Design review of the part built by this model. Coordinates are the model's own, in mm. Give positions to 0.01 mm unless a question says otherwise; leave off trailing zeros. Write each loop counter-clockwise with the first axis right and the second up, starting at its lowest first coordinate (ties: lowest second). Pieces come first, ordered by that corner, then holes. Notation, with made-up numbers: (2.25, 6.25) -> (29.25, 6.25) arc R12 ccw to (29.25, 12.25) -> close; hole circle Ø6 at (40.25, 39.25). An arc over 180 degrees is marked (long way). Put each result on its own line as item: value. Start each with the question number.
Autodesk Inventor part; units mm, degrees
ref_plane "YZ Plane" through (0, 0, 0) normal (1, 0, 0) x (0, 1, 0)
ref_plane "XZ Plane" through (0, 0, 0) normal (0, 1, 0) x (-1, 0, 0)
ref_plane "XY Plane" through (0, 0, 0) normal (0, 0, 1) x (1, 0, 0)
sketch "Sketch1" plane through (0, 0, 0) normal (0, 0, 1) x (1, 0, 0)
  line L0 (0, 0) -> (400, 0)
  line L1 (400, 0) -> (400, 100)
  line L2 (400, 100) -> (0, 100)
  line L3 (0, 100) -> (0, 0)
  line L4 (400, 100) -> (451.0344, 100) construction
  line L5 (0, 100) -> (51.0344, 100) construction
  line L6 (400, 100) -> (900.4511, 0)
  line L7 (400, 100) -> (910.3443, 100) construction
  line L8 (900.4511, 0) -> (400, 0)
  line L9 (0, 100) -> (-500.4511, 0)
  line L10 (0, 100) -> (510.3443, 100) construction
  line L11 (-500.4511, 0) -> (0, 0)
  dimension "d0" = 400
  dimension "d1" = 100
  dimension "d6" = 11.3
  dimension "d7" = 168.7
extrude "Extrusion1" add sketch "Sketch1" along normal blind 460
sketch "Sketch2" plane through (0, 100, 0) normal (0, 1, 0) x (1, 0, 0)
  line L0 (400, 0) -> (400, -460)
  line L1 (0, 0) -> (400, 0)
  line L2 (400, 0) -> (400, -30)
  line L3 (400, -30) -> (0, -30)
  line L4 (0, -30) -> (0, 0)
  line L5 (0, 0) -> (0, -460)
  line L6 (400, -460) -> (0, -460)
  line L7 (0, -460) -> (0, -430)
  line L8 (0, -430) -> (400, -430)
  line L9 (400, -430) -> (400, -460)
  dimension "d8" = 30
  dimension "d9" = 30
extrude "Extrusion2" add sketch "Sketch2" along normal blind 0.5 contours L0 L3 L4 L1 | L0 L6 L5 L8
sketch "Sketch3" plane through (900.4511, 0, 460) normal (0.1959, 0.9806, 0) x (0.9806, -0.1959, 0)
  line L0 (-1373.7453, 460) -> (0, 460)
  line L1 (-510.3443, 430) -> (-902.5902, 430)
  line L2 (0, 460) -> (-510.3443, 460)
  line L3 (-510.3443, 460) -> (-510.3443, 430)
  line L4 (-510.3443, 430) -> (0, 430)
  line L5 (0, 430) -> (0, 460)
  line L6 (0, 460) -> (0, 0)
  line L7 (-510.3443, 430) -> (-510.3443, 30)
  line L8 (0, 0) -> (-510.3443, 0)
  line L9 (-510.3443, 0) -> (-510.3443, 30)
  line L10 (-510.3443, 30) -> (0, 30)
  line L11 (0, 30) -> (0, 0)
  point P0 (-882.9956, 460)
  point P1 (-510.3443, 460)
  dimension "d12" = 30
  dimension "d13" = 510.3443
  dimension "d14" = 30
extrude "Extrusion3" add sketch "Sketch3" along normal blind 0.5 contours L0 L5 L4 L3 | L10 L6 L8 L9
sketch "Sketch4" plane through (-500.4511, 0, 460) normal (-0.1959, 0.9806, 0) x (0.9806, 0.1959, 0)
  line L0 (510.3443, 460) -> (0, 460)
  line L1 (902.5902, 430) -> (510.3443, 430)
  line L2 (0, 460) -> (510.3443, 460)
  line L3 (510.3443, 460) -> (510.3443, 430)
  line L4 (510.3443, 430) -> (0, 430)
  line L5 (0, 430) -> (0, 460)
  line L6 (510.3443, 0) -> (0, 0)
  line L7 (510.3443, 30) -> (902.5902, 30)
  line L8 (0, 0) -> (510.3443, 0)
  line L9 (510.3443, 0) -> (510.3443, 30)
  line L10 (510.3443, 30) -> (0, 30)
  line L11 (0, 30) -> (0, 0)
  point P0 (490.7497, 460)
  dimension "d17" = 30
  dimension "d18" = 30
extrude "Extrusion4" add sketch "Sketch4" along normal blind 0.5
sketch "Sketch5" plane through (0, 0, 0) normal (0, 0, -1) x (-1, 0, 0)
  line L0 (0, 100.5) -> (-400, 100.5)
  line L1 (500.5491, 0.4903) -> (0.098, 100.4903)
  line L2 (0, 100.5) -> (0.098, 100.4903)
  line L3 (500.4511, 0) -> (0, 100)
  line L4 (0.098, 100.4903) -> (0, 100)
  line L5 (0, 100) -> (0, 100.5)
  line L6 (0, 100) -> (0, 100.5)
  point P0 (0, 0)
extrude "Extrusion5" add sketch "Sketch5" against normal blind 460
sketch "Sketch6" plane through (0, 0, 0) normal (0, 0, -1) x (-1, 0, 0)
  line L0 (-400, 100) -> (-400, 100.5)
  line L1 (-400, 100.5) -> (-400, 100)
  line L2 (-400.098, 100.4903) -> (-900.5491, 0.4903)
  line L3 (-400, 100) -> (-400.098, 100.4903)
  line L4 (-400, 100.5) -> (0, 100.5)
  line L5 (-400.098, 100.4903) -> (-400, 100.5)
  point P0 (0, 0)
extrude "Extrusion6" add sketch "Sketch6" against normal blind 460
properties part number "cad bestanden"
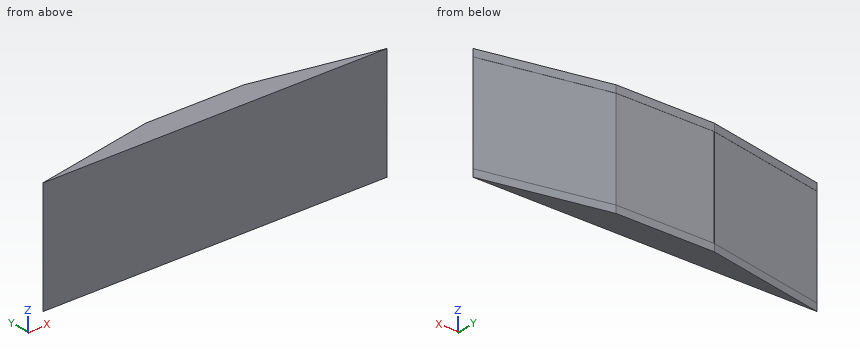
Q1. Take a section at C-C on y = 45.5. Give the boundary of the cut face in (x, z).
Q2. To check wall thickness, follow probe 1 along Y at (x, z) = (11, 229.5); probe 2 along Y at (x, z) = (696, 160.5). State the ranges of each line that lie inside material, in increasing order. Write a range as from..to.
Q3. Take a section at D-D on x = 656.5. Give the boundary of the cut face in (y, z).
Q4. Take a section at B-B on x = -288.5. Give the boundary of the cut face in (y, z), then the cut area to 3 significant figures.
Q5. For pin 1 (5 mm diameter, centred on x = 717, z = 79.5, fed in from +Y); pin 2 (10 mm diameter, centred on x = 211, z = 162, fed in from +Y), all flat-tipped, find the tip position at first contact; note any pin that passes through.
Result:
1. outline: (-275.25, 0) -> (675.25, 0) -> (675.25, 30) -> (672.75, 30) -> (672.75, 430) -> (675.25, 430) -> (675.25, 460) -> (-275.25, 460) -> (-275.25, 430) -> (-272.75, 430) -> (-272.75, 30) -> (-275.25, 30) -> close
2. probe 1: y = 0..100
2. probe 2: y = 0..40.85
3. outline: (0, 0) -> (49.25, 0) -> (49.25, 30) -> (48.75, 30) -> (48.75, 430) -> (49.25, 430) -> (49.25, 460) -> (0, 460) -> close
4. outline: (0, 0) -> (42.85, 0) -> (42.85, 30) -> (42.35, 30) -> (42.35, 430) -> (42.85, 430) -> (42.85, 460) -> (0, 460) -> close
4. area: 19,500 mm^2
5. pin 1: stops at y = 37.16
5. pin 2: stops at y = 100
